Here's how the part is built. I have some questions about the finished solid (model axes, mm). Face numbers are marked on the shaded views. Give positions to 0.01 mm unless a question says otherwise; leave off trailing zeros. Write each loop counter-clockwise with the first axis right and the second up, starting at its lowest first coordinate (ties: lowest second). Pieces come first, ordered by that corner, then holes. Notation, with made-up numbers: (58.25, 2.25) -> (104.25, 2.25) arc R6 cw to (104.25, 11.25) -> close; hole circle Ø7 at (79.25, 46.5). An arc over 180 degrees is marked (long way). Use one line per item in the form item = value.
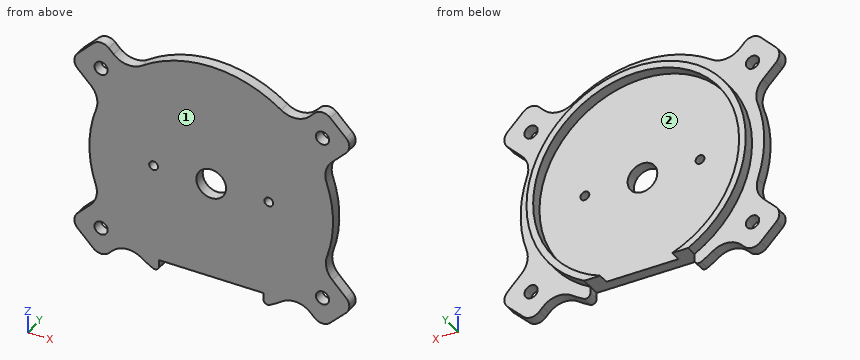
```python
from build123d import *

# Parameters (mm, degrees)
SKETCH_1_R                  = 55
EXTRUDE_1_DEPTH             = 5
SKETCH_5_W                  = 47
SKETCH_5_H                  = 12.24289715
CUT_EXTRUDE_2_DEPTH         = 30
FILLET_4_R                  = 2
FILLET_5_R                  = 2
EXTRUDE_3_REACH             = 79.84
EXTRUDE_3_DIRECTION_2_REACH = 79.84
FILLET_7_R                  = 10
FILLET_8_R                  = 5
SKETCH_10_R                 = 3
CUT_EXTRUDE_5_DEPTH         = 5
SKETCH_15_R                 = 6.7
CUT_EXTRUDE_6_DEPTH         = 10
SKETCH_16_R                 = 2
CUT_EXTRUDE_7_DEPTH         = 10
EXTRUDE_4_DEPTH             = 5


with BuildPart() as part:
    # 草图1 → 凸台-拉伸1 (new body)
    with BuildSketch(Plane(origin=(0, 0, 0), x_dir=(1, 0, 0), z_dir=(0, 1, 0))):
        with Locations(Location((0, 0, 0), (0, 0, 270))):
            Circle(SKETCH_1_R)
    extrude(amount=EXTRUDE_1_DEPTH)

    # 草图5 → 切除-拉伸2 (cut)
    with BuildSketch(Plane(origin=(0, 5, 0), x_dir=(1, 0, 0), z_dir=(0, 1, 0))):
        with Locations((0, 49.687490397)):
            Rectangle(SKETCH_5_W, SKETCH_5_H)
    extrude(amount=-CUT_EXTRUDE_2_DEPTH, mode=Mode.SUBTRACT)

    # 圆角4
    fillet_4_edges = [part.edges().sort_by_distance(p)[0] for p in [
        (-23.5, 2.5, -49.726753363),
    ]]
    fillet(fillet_4_edges, radius=FILLET_4_R)

    # 圆角5
    fillet_5_edges = [part.edges().sort_by_distance(p)[0] for p in [
        (23.5, 2.5, -49.726753363),
    ]]
    fillet(fillet_5_edges, radius=FILLET_5_R)

    # 凸台-拉伸3: up to this face of the body (flat: up to its plane)
    extrude_3_end = Plane(part.part.faces().sort_by_distance((0, 0, 2.477505486))[0])
    # 草图14 → 凸台-拉伸3 (add, up to the picked face)
    with BuildSketch(Plane(origin=(0, 3, 0), x_dir=(1, 0, 0), z_dir=(0, 1, 0)), mode=Mode.PRIVATE) as extrude_3_sk1:
        with BuildLine():
            Line((-49.898576095, 23.132922507), (-63.862525635, 37.044772973))
            Line((-63.862525635, 37.044772973), (-49.746845912, 51.213315099))
            Line((-49.746845912, 51.213315099), (-38.128637352, 39.638453724))
            ThreePointArc((-38.128637352, 39.638453724), (-44.78063998, 31.932652301), (-49.898576095, 23.132922507))
        make_face()
    extrude_3_tool1 = split(extrude(extrude_3_sk1.sketch, amount=-EXTRUDE_3_REACH, mode=Mode.PRIVATE), bisect_by=extrude_3_end, keep=Keep.BOTH, mode=Mode.PRIVATE)
    # 草图14 → 凸台-拉伸3 (add, up to the picked face)
    with BuildSketch(Plane(origin=(0, 3, 0), x_dir=(1, 0, 0), z_dir=(0, 1, 0)), mode=Mode.PRIVATE) as extrude_3_sk2:
        with BuildLine():
            Line((49.811900188, -23.3189751), (64.421720913, -37.928795825))
            Line((64.421720913, -37.928795825), (50.279585289, -52.070931449))
            Line((50.279585289, -52.070931449), (37.984884655, -39.776230814))
            ThreePointArc((37.984884655, -39.776230814), (44.662950793, -32.097053236), (49.811900188, -23.3189751))
        make_face()
    extrude_3_tool2 = split(extrude(extrude_3_sk2.sketch, amount=-EXTRUDE_3_REACH, mode=Mode.PRIVATE), bisect_by=extrude_3_end, keep=Keep.BOTH, mode=Mode.PRIVATE)
    # 草图14 → 凸台-拉伸3 (add, up to the picked face)
    with BuildSketch(Plane(origin=(0, 3, 0), x_dir=(1, 0, 0), z_dir=(0, 1, 0)), mode=Mode.PRIVATE) as extrude_3_sk3:
        with BuildLine():
            Line((-49.632393674, -23.698639164), (-63.862550335, -37.928795825))
            Line((-63.862550335, -37.928795825), (-49.720414711, -52.070931449))
            Line((-49.720414711, -52.070931449), (-37.697852746, -40.048369484))
            ThreePointArc((-37.697852746, -40.048369484), (-44.423770724, -32.427281642), (-49.632393674, -23.698639164))
        make_face()
    extrude_3_tool3 = split(extrude(extrude_3_sk3.sketch, amount=-EXTRUDE_3_REACH, mode=Mode.PRIVATE), bisect_by=extrude_3_end, keep=Keep.BOTH, mode=Mode.PRIVATE)
    # 草图14 → 凸台-拉伸3 (add, up to the picked face)
    with BuildSketch(Plane(origin=(0, 3, 0), x_dir=(1, 0, 0), z_dir=(0, 1, 0)), mode=Mode.PRIVATE) as extrude_3_sk4:
        with BuildLine():
            Line((38.475737251, 39.301623923), (50.118901666, 51.212426922))
            Line((50.118901666, 51.212426922), (64.420808036, 37.231887798))
            Line((64.420808036, 37.231887798), (50.134465219, 22.6171483))
            ThreePointArc((50.134465219, 22.6171483), (45.083643676, 31.50341367), (38.475737251, 39.301623923))
        make_face()
    extrude_3_tool4 = split(extrude(extrude_3_sk4.sketch, amount=-EXTRUDE_3_REACH, mode=Mode.PRIVATE), bisect_by=extrude_3_end, keep=Keep.BOTH, mode=Mode.PRIVATE)
    add(extrude_3_tool1.solids().sort_by(Axis((-50.837096, 3, -37.73966), (0, -1, 0)))[0])
    add(extrude_3_tool2.solids().sort_by(Axis((51.039653, 3, 38.272151), (0, -1, 0)))[0])
    add(extrude_3_tool3.solids().sort_by(Axis((-50.639154, 3, 38.439997), (0, -1, 0)))[0])
    add(extrude_3_tool4.solids().sort_by(Axis((51.238479, 3, -37.552164), (0, -1, 0)))[0])

    # 凸台-拉伸3 direction 2: up to this face of the body (flat: up to its plane)
    extrude_3_direction_2_end = Plane(part.part.faces().sort_by_distance((0, 5, 2.477505486))[0])
    # 草图14 → 凸台-拉伸3 direction 2 (add, up to the picked face)
    with BuildSketch(Plane(origin=(0, 3, 0), x_dir=(1, 0, 0), z_dir=(0, 1, 0)), mode=Mode.PRIVATE) as extrude_3_direction_2_sk1:
        with BuildLine():
            Line((-49.898576095, 23.132922507), (-63.862525635, 37.044772973))
            Line((-63.862525635, 37.044772973), (-49.746845912, 51.213315099))
            Line((-49.746845912, 51.213315099), (-38.128637352, 39.638453724))
            ThreePointArc((-38.128637352, 39.638453724), (-44.78063998, 31.932652301), (-49.898576095, 23.132922507))
        make_face()
    extrude_3_direction_2_tool1 = split(extrude(extrude_3_direction_2_sk1.sketch, amount=EXTRUDE_3_DIRECTION_2_REACH, mode=Mode.PRIVATE), bisect_by=extrude_3_direction_2_end, keep=Keep.BOTH, mode=Mode.PRIVATE)
    # 草图14 → 凸台-拉伸3 direction 2 (add, up to the picked face)
    with BuildSketch(Plane(origin=(0, 3, 0), x_dir=(1, 0, 0), z_dir=(0, 1, 0)), mode=Mode.PRIVATE) as extrude_3_direction_2_sk2:
        with BuildLine():
            Line((49.811900188, -23.3189751), (64.421720913, -37.928795825))
            Line((64.421720913, -37.928795825), (50.279585289, -52.070931449))
            Line((50.279585289, -52.070931449), (37.984884655, -39.776230814))
            ThreePointArc((37.984884655, -39.776230814), (44.662950793, -32.097053236), (49.811900188, -23.3189751))
        make_face()
    extrude_3_direction_2_tool2 = split(extrude(extrude_3_direction_2_sk2.sketch, amount=EXTRUDE_3_DIRECTION_2_REACH, mode=Mode.PRIVATE), bisect_by=extrude_3_direction_2_end, keep=Keep.BOTH, mode=Mode.PRIVATE)
    # 草图14 → 凸台-拉伸3 direction 2 (add, up to the picked face)
    with BuildSketch(Plane(origin=(0, 3, 0), x_dir=(1, 0, 0), z_dir=(0, 1, 0)), mode=Mode.PRIVATE) as extrude_3_direction_2_sk3:
        with BuildLine():
            Line((-49.632393674, -23.698639164), (-63.862550335, -37.928795825))
            Line((-63.862550335, -37.928795825), (-49.720414711, -52.070931449))
            Line((-49.720414711, -52.070931449), (-37.697852746, -40.048369484))
            ThreePointArc((-37.697852746, -40.048369484), (-44.423770724, -32.427281642), (-49.632393674, -23.698639164))
        make_face()
    extrude_3_direction_2_tool3 = split(extrude(extrude_3_direction_2_sk3.sketch, amount=EXTRUDE_3_DIRECTION_2_REACH, mode=Mode.PRIVATE), bisect_by=extrude_3_direction_2_end, keep=Keep.BOTH, mode=Mode.PRIVATE)
    # 草图14 → 凸台-拉伸3 direction 2 (add, up to the picked face)
    with BuildSketch(Plane(origin=(0, 3, 0), x_dir=(1, 0, 0), z_dir=(0, 1, 0)), mode=Mode.PRIVATE) as extrude_3_direction_2_sk4:
        with BuildLine():
            Line((38.475737251, 39.301623923), (50.118901666, 51.212426922))
            Line((50.118901666, 51.212426922), (64.420808036, 37.231887798))
            Line((64.420808036, 37.231887798), (50.134465219, 22.6171483))
            ThreePointArc((50.134465219, 22.6171483), (45.083643676, 31.50341367), (38.475737251, 39.301623923))
        make_face()
    extrude_3_direction_2_tool4 = split(extrude(extrude_3_direction_2_sk4.sketch, amount=EXTRUDE_3_DIRECTION_2_REACH, mode=Mode.PRIVATE), bisect_by=extrude_3_direction_2_end, keep=Keep.BOTH, mode=Mode.PRIVATE)
    add(extrude_3_direction_2_tool1.solids().sort_by(Axis((-50.837096, 3, -37.73966), (0, 1, 0)))[0])
    add(extrude_3_direction_2_tool2.solids().sort_by(Axis((51.039653, 3, 38.272151), (0, 1, 0)))[0])
    add(extrude_3_direction_2_tool3.solids().sort_by(Axis((-50.639154, 3, 38.439997), (0, 1, 0)))[0])
    add(extrude_3_direction_2_tool4.solids().sort_by(Axis((51.238479, 3, -37.552164), (0, 1, 0)))[0])

    # 圆角7
    fillet_7_edges = [part.edges().sort_by_distance(p)[0] for p in [
        (-38.128637352, 2.5, -39.638453724),
        (-49.898576095, 2.5, -23.132922507),
        (-49.632393674, 2.5, 23.698639164),
        (-37.697852746, 2.5, 40.048369484),
        (50.134465219, 2.5, -22.6171483),
        (38.475737251, 2.5, -39.301623923),
        (37.984884655, 2.5, 39.776230814),
        (49.811900188, 2.5, 23.3189751),
    ]]
    fillet(fillet_7_edges, radius=FILLET_7_R)

    # 圆角8
    fillet_8_edges = [part.edges().sort_by_distance(p)[0] for p in [
        (-63.862525635, 2.5, -37.044772973),
        (-49.746845912, 2.5, -51.213315099),
        (-49.720414711, 2.5, 52.070931449),
        (-63.862550335, 2.5, 37.928795825),
        (50.118901666, 2.5, -51.212426922),
        (64.420808036, 2.5, -37.231887798),
        (50.279585289, 2.5, 52.070931449),
        (64.421720913, 2.5, 37.928795825),
    ]]
    fillet(fillet_8_edges, radius=FILLET_8_R)

    # 草图10 → 切除-拉伸5 (cut, symmetric)
    with BuildSketch(Plane(origin=(0, 3, 0), x_dir=(1, 0, 0), z_dir=(0, 1, 0))):
        with Locations(Location((-49.720414711, 37.071204175, 0), (0, 0, 270))):
            Circle(SKETCH_10_R)
        with Locations(Location((50.279585289, 37.071204175, 0), (0, 0, 270))):
            Circle(SKETCH_10_R)
        with Locations(Location((-49.720414711, -37.928795825, 0), (0, 0, 270))):
            Circle(SKETCH_10_R)
        with Locations(Location((50.279585289, -37.928795825, 0), (0, 0, 270))):
            Circle(SKETCH_10_R)
    extrude(amount=CUT_EXTRUDE_5_DEPTH, both=True, mode=Mode.SUBTRACT)

    # 草图15 → 切除-拉伸6 (cut)
    with BuildSketch(Plane(origin=(0, 5, 0), x_dir=(1, 0, 0), z_dir=(0, 1, 0))):
        with Locations(Location((0, 0, 0), (0, 0, 270))):
            Circle(SKETCH_15_R)
    extrude(amount=-CUT_EXTRUDE_6_DEPTH, mode=Mode.SUBTRACT)

    # 草图16 → 切除-拉伸7 (cut)
    with BuildSketch(Plane(origin=(0, 5, 0), x_dir=(1, 0, 0), z_dir=(0, 1, 0))):
        with Locations(Location((-26, 0, 0), (0, 0, 270))):
            Circle(SKETCH_16_R)
        with Locations(Location((26, 0, 0), (0, 0, 270))):
            Circle(SKETCH_16_R)
    extrude(amount=-CUT_EXTRUDE_7_DEPTH, mode=Mode.SUBTRACT)

    # 草图17 → 凸台-拉伸4 (add)
    with BuildSketch(Plane(origin=(0, 5, 0), x_dir=(1, 0, 0), z_dir=(0, 1, 0))):
        with BuildLine():
            Line((-23.5, 43.566041822), (-16.255768207, 43.566041822))
            ThreePointArc((-16.255768207, 43.566041822), (0, -46.5), (16.255768207, 43.566041822))
            Line((16.255768207, 43.566041822), (23.5, 43.566041822))
            ThreePointArc((23.5, 43.566041822), (0, -49.5), (-23.5, 43.566041822))
        make_face()
    extrude(amount=EXTRUDE_4_DEPTH)


solid = part.part
```
Q1. Will these pins go through, and if not, where does the flat tip stop? pin 1 Ø2 at (y, z) = (3.5, 29) entering from -X; pin 2 Ø5 at (x, z) = (-26, 0) entering from +Y; pin 3 Ø2 at (x, y) = (49, 4.5) entering from -Z.
Result set:
pin_1 = -55.93
pin_2 = 5
pin_3 = -49.14
Q2. If we mould it in two halves opening along Z, with no side actions, what happens to the marked faces 1 and 2? For each: +Z half, -Z half, draft (parallel to the pull), parting line (faces both ways), or undercut.
Result set:
face_1 = draft
face_2 = undercut
Q3. I want a section at D-D, the plane y = 3.25. Count the separate pieces of the cut face and the enclosed holes in it, and give its area (3 significant figures).
Result set:
separate_pieces = 1
enclosed_holes = 7
area = 10,200 mm2
Q4. I want a section at A-A, the plane x = 0. Write out the boundary of the cut face in (y, z), and give its area (3 significant figures).
Result set:
outline = (0, -43.57) -> (5, -43.57) -> (5, -6.7) -> (0, -6.7) -> close; (0, 6.7) -> (5, 6.7) -> (5, 46.5) -> (10, 46.5) -> (10, 49.5) -> (5, 49.5) -> (5, 55) -> (0, 55) -> close
area = 441 mm2
Q5. If I drill on line 1 along X through (y, z) = (3.6, 0); line 2 along Z through (x, y) = (0, 8.7); line 3 along X through (y, z) = (7, -39), over which ranges is the centre line in solid material (lowest first)? Write a range as from..to.
Result set:
line_1 = -55..-28, -24..-6.7, 6.7..24, 28..55
line_2 = 46.5..49.5
line_3 = -30.48..-25.32, 25.32..30.48
Q6. I want a section at C-C, the plane x = 38.5. Write out the boundary of the cut face in (y, z).
Result set:
outline = (0, -42.92) -> (5, -42.92) -> (5, -31.11) -> (10, -31.11) -> (10, -26.08) -> (5, -26.08) -> (5, 26.08) -> (10, 26.08) -> (10, 31.11) -> (5, 31.11) -> (5, 43.31) -> (0, 43.31) -> close
Q7. I want a section at B-B, the plane z = 9.5. Write out the boundary of the cut face in (x, y).
Result set:
outline = (-54.17, 0) -> (54.17, 0) -> (54.17, 5) -> (48.58, 5) -> (48.58, 10) -> (45.52, 10) -> (45.52, 5) -> (-45.52, 5) -> (-45.52, 10) -> (-48.58, 10) -> (-48.58, 5) -> (-54.17, 5) -> close
